```python
from build123d import *

# Parameters (mm, degrees)
F1_DEPTH = 63.5
F0_W     = 25.1397234082
F0_H     = 19.05
F2_DEPTH = 25.4
F3_DEPTH = 7.9375


with BuildPart() as f1:
    # F0 (on Front) → F1 (new body, symmetric)
    with BuildSketch(Plane.XZ):
        Polygon((-41.275, 9.525), (-41.275, -9.525), (41.275, -9.525), (41.275, 9.525), (22.225, 9.525), align=None)
    extrude(amount=F1_DEPTH, both=True)

    # F0 (on Front) → F2 (join, symmetric)
    with BuildSketch(Plane.XZ):
        with BuildLine():
            Line((22.225, 9.525), (41.275, 9.525))
            Line((41.275, 9.525), (41.275, 27.0002))
            ThreePointArc((41.275, 27.0002), (45.9246798487, 38.2255201513), (57.15, 42.8752))
            Line((57.15, 42.8752), (60.325, 42.8752))
            Line((60.325, 42.8752), (60.325, 61.9252))
            Line((60.325, 61.9252), (57.15, 61.9252))
            ThreePointArc((57.15, 61.9252), (32.4542956671, 51.6959043329), (22.225, 27.0002))
            Line((22.225, 27.0002), (22.225, 9.525))
        make_face()
        with Locations((72.8948617041, 52.4002)):
            Rectangle(F0_W, F0_H)
    extrude(amount=F2_DEPTH, both=True)

    # F0 (on Front) → F3 (join, symmetric)
    with BuildSketch(Plane.XZ):
        with BuildLine():
            add(Edge.make_bspline(
                [(-41.275, 9.525), (-41.275, 42.1362832522), (18.6590275409, 61.9252), (57.15, 61.9252)],
                knots=[0, 0, 0, 0, 111.5045361635, 111.5045361635, 111.5045361635, 111.5045361635], degree=3))
            Line((-41.275, 9.525), (22.225, 9.525))
            Line((22.225, 9.525), (22.225, 27.0002))
            ThreePointArc((22.225, 27.0002), (32.4542956671, 51.6959043329), (57.15, 61.9252))
        make_face()
    extrude(amount=F3_DEPTH, both=True)

    # F0 (on Front) → F4 (revolve)
    with BuildSketch(Plane.XZ):
        Polygon((111.125, 66.675), (85.725, 66.675), (85.4647234082, 38.1), (111.125, 38.1), align=None)
    revolve(axis=Axis((85.5948617041, 0, 52.3875), (-0.0091081643, 0, -0.9999585198)))


solid = f1.part
```
CAD build for the part. Positions are in the model's coordinates, mm. A direction names the side the tool comes from. Give positions to 0.01 mm unless a question says otherwise; leave off trailing zeros. Order: outer loops, then holes, each group sorted by start corner. A loop starts at its lowest first (then second) coordinate and runs counter-clockwise, first axis right, second up.
(1) Flat gauge pins, fed straight in: pin 1 (18.5 mm diameter, centred on y = 23.5, z = 0, fed in from +X) (3 decimals); pin 2 (8 mm diameter, centred on x = 74, z = 40, fed in from +Y); pin 3 (12.5 mm diameter, centred on x = 70, y = 10.5, fed in from -Z). Where does each tip first touch, or does it go through?
(2) Mould opens along X. For faces 1 (the conical face through (86.9, 0.6, 38.1)), 2 (the flat face through (-2, 7.938, 30)), 3 (the cylindrical face through (32.73, 16.55, 51.97)) say: released by +X, released by -X, zero draft, split by the parting line, or undercut.
(3) Tool access for faces 4 (the cylindrical face through (45.8, -0.4, 38.1)), 5 (the conical face through (86.901, -0.37, 66.676)), 6 (the flat face through (60, 0, 61.925)), 7 (the flat face through (22.225, -17, 18)), 8 (the flat face through (22.225, 17, 18)): list every direction of +Z, -Z, +X, -X, +Y, -Y with a clear straight run to the whole face (end or side of a thin tool).
(4) Drill centre lines: L1, parallel to Z at x = 12, y = -51.5 (3 decimals); L2, parallel to Y at x = -16, z = 24; L3, parallel to X at y = -16.5, z = 2 (3 decimals). Where is each one in solid material? Low to high.
(5) Saw through at B-B, the plane z = 0.5. Give the cut face in (x, y) (3 decimals).
(6) Saw through at A-A, the plane y = 53.5. Give the cut face in (x, z) (3 decimals).
Results found:
1. pin 1: stops at x = 41.275
1. pin 2: stops at y = 25.4
1. pin 3: stops at z = 38.3
2. face 1: undercut
2. face 2: zero draft
2. face 3: released by -X
3. face 4: -Z, +Y, -Y
3. face 5: +Z, +X
3. face 6: +Z, -X
3. face 7: +Z, -X, -Y
3. face 8: +Z, -X, +Y
4. L1: z = -9.525 to 9.525
4. L2: y = -7.94 to 7.94
4. L3: x = -41.275 to 41.275
5. outline: (-41.275, -63.5) - (41.275, -63.5) - (41.275, 63.5) - (-41.275, 63.5) - close
6. outline: (-41.275, -9.525) - (41.275, -9.525) - (41.275, 9.525) - (-41.275, 9.525) - close
